Build history of the part. All positions in model axes, mm. Face numbers are marked on the shaded views. A direction names the side the tool comes from. Round coordinates to 2 decimals unless told otherwise and drop trailing zeros. Order: outer loops, then holes, each group sorted by start corner. A loop starts at its lowest first (then second) coordinate and runs counter-clockwise, first axis right, second up. Notation, with made-up numbers: (5.25, -12) -> (38.25, -12) arc R34 cw to (38.25, 23) -> close; hole circle Ø7 at (77.25, -2.75). An arc over 180 degrees is marked (long way). Use a Markdown table: item, result. Add a question column.
Item 1: Two-plate mould, pull along X, no slides. Class the marked faces 4, 5, 6 and 7: released by +X, released by -X, zero draft, split by the parting line, or undercut.
Item 2: Probe L1, parallel to Y at x = 38.75, z = 0 (3 decimals); L2, parallel to Z at x = 35, y = 4 (3 decimals); L3, parallel to X at y = 5.5, z = -39. List the from-to ranges inside material, lowest first.
Item 3: 3-axis set-ups, long thin cutter, end or side, ignore diameter. For the marked faces 1, 2 and 3: which of +Z, -Z, +X, -X, +Y, -Y reach the whole face in a straight line?
Item 4: Slice it at D-D, the plane z = 0. Give the cut face in (x, y) (3 decimals).
Item 5: Pin check, flat tips, straight feed: pin 1 (6 mm diameter, centred on y = 11, z = -24, fed in from +X); pin 2 (1 mm diameter, centred on y = 8, z = -6.5, fed in from +X); pin 3 (7.5 mm diameter, centred on y = 3.5, z = -0.5, fed in from -X); pin 4 (3.5 mm diameter, centred on x = -1.5, y = 8.5, fed in from -Z). Stop position of each tip, or through.
Item 6: Slice it at C-C, the plane x = -17.5. Give the cut face in (y, z), plus the area to 3 significant figures.
Item 7: Slice it at B-B, the plane y = 16.25. Give the cut face in (x, z).
Item 8: Slice it at A-A, the plane z = -31.5. Give the cut face in (x, y).
from build123d import *

# Parameters (mm, degrees)
SKETCH1_W           = 64
SKETCH1_H           = 40
BOSS_EXTRUDE1_DEPTH = 12
SKETCH2_R           = 5
SKETCH2_R_2         = 3.515
BOSS_EXTRUDE2_DEPTH = 13
BOSS_EXTRUDE3_START = 13
SKETCH3_R           = 5
SKETCH3_R_2         = 3.515
BOSS_EXTRUDE3_DEPTH = 13
SKETCH5_W           = 10
SKETCH5_H           = 10
BOSS_EXTRUDE4_DEPTH = 22
SKETCH6_W           = 10
SKETCH6_H           = 2
BOSS_EXTRUDE5_DEPTH = 10


with BuildPart() as part:
    # Sketch1 → Boss-Extrude1 (new body)
    with BuildSketch(Plane(origin=(0, 0, 0), x_dir=(1, 0, 0), z_dir=(0, 1, 0))):
        Rectangle(SKETCH1_W, SKETCH1_H)
    extrude(amount=BOSS_EXTRUDE1_DEPTH)

    # Sketch2 → Boss-Extrude2 (add)
    with BuildSketch(Plane(origin=(32, 0, 0), x_dir=(0, 0, -1), z_dir=(1, 0, 0))):
        with Locations(Location((0, 4, 0), (0, 0, 233.130102354))):
            Circle(SKETCH2_R)
        with Locations(Location((0, 4, 0), (0, 0, 180))):
            Circle(SKETCH2_R_2, mode=Mode.SUBTRACT)
    extrude(amount=BOSS_EXTRUDE2_DEPTH)

    # Sketch3 → Boss-Extrude3 (add)
    with BuildSketch(Plane.ZY.offset(32).offset(BOSS_EXTRUDE3_START)):
        with Locations(Location((0, 4, 0), (0, 0, 306.869897646))):
            Circle(SKETCH3_R)
        with Locations((0, 4)):
            Circle(SKETCH3_R_2, mode=Mode.SUBTRACT)
    extrude(amount=-BOSS_EXTRUDE3_DEPTH)

    # Sketch5 → Boss-Extrude4 (add)
    with BuildSketch(Plane(origin=(0, 0, -20), x_dir=(-1, 0, 0), z_dir=(0, 0, -1))):
        with Locations((-20, 6)):
            Rectangle(SKETCH5_W, SKETCH5_H)
        with Locations((20, 6)):
            Rectangle(SKETCH5_W, SKETCH5_H)
    extrude(amount=BOSS_EXTRUDE4_DEPTH)

    # Sketch6 → Boss-Extrude5 (add)
    with BuildSketch(Plane(origin=(0, 11, 0), x_dir=(1, 0, 0), z_dir=(0, 1, 0))):
        with Locations((20, 41)):
            Rectangle(SKETCH6_W, SKETCH6_H)
        with Locations((-20, 41)):
            Rectangle(SKETCH6_W, SKETCH6_H)
    extrude(amount=BOSS_EXTRUDE5_DEPTH)


solid = part.part
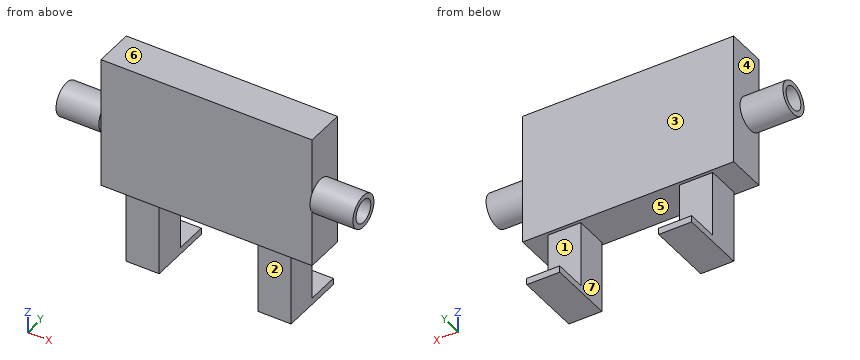
Check sheet entries:
| question | item | result |
|---|---|---|
| 1 | face 4 | released by -X |
| 1 | face 5 | undercut |
| 1 | face 6 | zero draft |
| 1 | face 7 | undercut |
| 2 | L1 | -1 to 0.485, 7.515 to 9 |
| 2 | L2 | -5 to -3.515, 3.515 to 5 |
| 2 | L3 | -25 to -15, 15 to 25 |
| 3 | face 1 | +X, -X, +Y |
| 3 | face 2 | -Z, +X, -X, -Y |
| 3 | face 3 | +Z, +X, -X, +Y |
| 4 | outline | (-45, -1) -> (-32, -1) -> (-32, 0) -> (32, 0) -> (32, -1) -> (45, -1) -> (45, 0.485) -> (32, 0.485) -> (32, 7.515) -> (45, 7.515) -> (45, 9) -> (32, 9) -> (32, 12) -> (-32, 12) -> (-32, 9) -> (-45, 9) -> (-45, 7.515) -> (-32, 7.515) -> (-32, 0.485) -> (-45, 0.485) -> close |
| 5 | pin 1 | x = 25 |
| 5 | pin 2 | x = 32 |
| 5 | pin 3 | x = -45 |
| 5 | pin 4 | z = -20 |
| 6 | outline | (0, -20) -> (1, -20) -> (1, -42) -> (21, -42) -> (21, -40) -> (11, -40) -> (11, -20) -> (12, -20) -> (12, 20) -> (0, 20) -> close |
| 6 | area | 720 mm2 |
| 7 | outline | (-25, -42) -> (-15, -42) -> (-15, -40) -> (-25, -40) -> close; (15, -42) -> (25, -42) -> (25, -40) -> (15, -40) -> close |
| 8 | outline | (-25, 1) -> (-15, 1) -> (-15, 11) -> (-25, 11) -> close; (15, 1) -> (25, 1) -> (25, 11) -> (15, 11) -> close |
